Drawing for the job (mm, zero at the part's lowest x, y, z). A direction names the side the tool comes from. Give positions to 0.01 mm unless a question says otherwise; leave off trailing zeros. Loops run counter-clockwise (first coordinate to the right, second up) from the corner with the lowest first, then second, coordinate; pieces in that order, holes last. Notation, with made-up numbers: (36, -35) -> (46, -35) arc R32 ccw to (46, -1) -> close; hole circle Ø10 at (36, -24.75). An arc over 180 degrees is marked (long way). Write item = value, one per line.
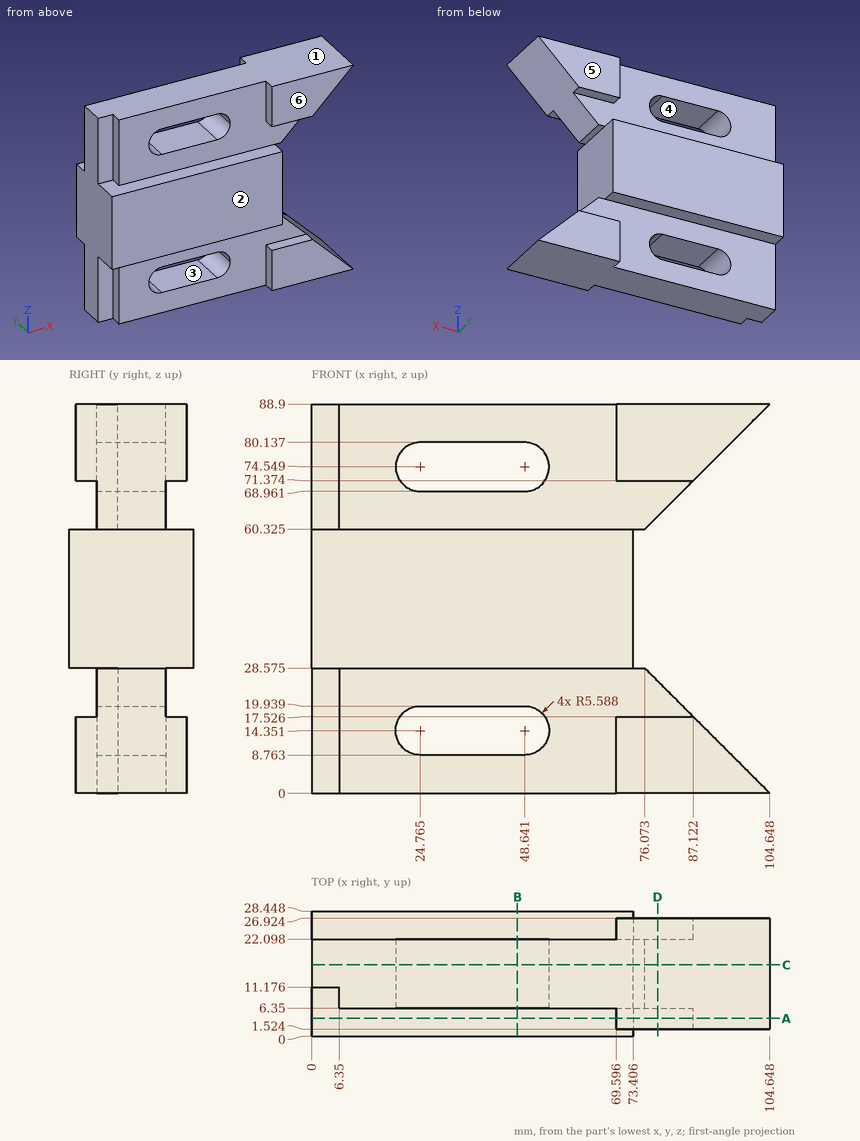
1) Slice it at C-C, the plane y = 16.25. List the corners of the cut face in (x, z) (3 decimals).
Resolved:
outline = (0, 0) -> (104.648, 0) -> (76.073, 28.575) -> (73.406, 28.575) -> (73.406, 60.325) -> (76.073, 60.325) -> (104.648, 88.9) -> (0, 88.9) -> close; hole (24.765, 8.763) -> (48.641, 8.763) arc R5.588 ccw to (54.229, 14.351) arc R5.588 ccw to (48.641, 19.939) -> (24.765, 19.939) arc R5.588 ccw to start; hole (24.765, 68.961) -> (48.641, 68.961) arc R5.588 ccw to (54.229, 74.549) arc R5.588 ccw to (48.641, 80.137) -> (24.765, 80.137) arc R5.588 ccw to start
2) Slice it at B-B, the plane x = 47. List the corners of the cut face in (y, z) (3 decimals).
Resolved:
outline = (0, 28.575) -> (6.35, 28.575) -> (6.35, 19.939) -> (22.098, 19.939) -> (22.098, 28.575) -> (28.448, 28.575) -> (28.448, 60.325) -> (22.098, 60.325) -> (22.098, 68.961) -> (6.35, 68.961) -> (6.35, 60.325) -> (0, 60.325) -> close; (6.35, 0) -> (22.098, 0) -> (22.098, 8.763) -> (6.35, 8.763) -> close; (6.35, 80.137) -> (22.098, 80.137) -> (22.098, 88.9) -> (6.35, 88.9) -> close
3) Slice it at D-D, the plane x = 79. List the corners of the cut face in (y, z), and give its area (3 significant figures).
Resolved:
outline = (1.52, 0) -> (26.92, 0) -> (26.92, 17.53) -> (22.1, 17.53) -> (22.1, 25.65) -> (6.35, 25.65) -> (6.35, 17.53) -> (1.52, 17.53) -> close; (1.52, 71.37) -> (6.35, 71.37) -> (6.35, 63.25) -> (22.1, 63.25) -> (22.1, 71.37) -> (26.92, 71.37) -> (26.92, 88.9) -> (1.52, 88.9) -> close
area = 1,150 mm²
4) Drill centre lines: line 1 along Z through (x, y) = (47, 17); line 2 along Z through (x, y) = (51, 15.25); line 3 along Y through (x, z) = (60.5, 13.5). Where is each one in solid material? Low to high. Write a range as [from, to].
Resolved:
line_1 = [0, 8.76], [19.94, 68.96], [80.14, 88.9]
line_2 = [0, 9.29], [19.42, 69.48], [79.61, 88.9]
line_3 = [6.35, 22.1]
5) Drop flat-ended pins along their axis: P1, Ø7, axis at x = 2, z = 11, coming from the -Y side; P2, Ø3.5, axis at x = 40.5, y = 4.5, coming from the +Z side (3 decimals); P3, Ø10, axis at x = 65.5, z = 10, coming from the +Y side. Give the stop position or say it passes through.
Resolved:
P1 = 11.18
P2 = 60.325
P3 = 26.92
6) Pull direction Z, two halves, no side cores. Call the marked faces 1, 2 and 3: pulls with the +Z half, pulls with the -Z half, needs draft (parallel to the pull), parting line crosses it, or undercut.
Resolved:
face_1 = pulls with the +Z half
face_2 = needs draft
face_3 = undercut
7) Slice it at A-A, the plane y = 4. List the corners of the cut face in (x, z) (3 decimals).
Resolved:
outline = (0, 28.575) -> (73.406, 28.575) -> (73.406, 60.325) -> (0, 60.325) -> close; (69.596, 0) -> (104.648, 0) -> (87.122, 17.526) -> (69.596, 17.526) -> close; (69.596, 71.374) -> (87.122, 71.374) -> (104.648, 88.9) -> (69.596, 88.9) -> close
8) Which spindle directions (+Z, -Z, +X, -X, +Y, -Y) get a long thin tool onto all of the face, cutting with end or side? Do the marked faces 4, 5 and 6. Say none if no direction does.
Resolved:
face_4 = +Y, -Y
face_5 = +Z, +X, -X, +Y
face_6 = +Z, +X, -X, -Y
